Could you check a few things on this model? Use its own coordinates, in mm. A direction names the side the tool comes from. Round coordinates to 2 decimals unless told otherwise and drop trailing zeros. Loops run counter-clockwise (first coordinate to the right, second up) from the corner with the lowest first, then second, coordinate; pieces in that order, holes last.
Autodesk Inventor part; units mm, degrees
ref_plane "Plano de trabajo1" through (0, 91.5, 0) normal (0, 1, 0) x (1, 0, 0)
ref_plane "YZ Plane" through (0, 0, 0) normal (1, 0, 0) x (0, 1, 0)
ref_plane "XZ Plane" through (0, 0, 0) normal (0, 1, 0) x (-1, 0, 0)
sketch "Boceto1" plane through (0, 0, 0) normal (0, 1, 0) x (-1, 0, 0)
  circle A0 centre (0, 0) radius 11
  dimension "d0" = 22
extrude "Extrusión1" add sketch "Boceto1" along normal blind 105
ref_plane "Plano de trabajo1" through (0, 91.5, 0) normal (0, 1, 0) x (1, 0, 0)
sketch "Boceto2" plane through (0, 91.5, 0) normal (0, 1, 0) x (1, 0, 0)
  circle A0 centre (0, 0) radius 11
  circle A1 centre (0, 0) radius 10
  dimension "d4" = 20
extrude "Extrusión2" cut sketch "Boceto2" against normal blind 1
thread "Rosca1"
properties part number "W520superior"
Item 1: For faces 5 (the flat face through (2, 90.5, 10)), 6 (the cylindrical face through (2.38, 98.16, 10.74)), which set-ups out of +Z, -Z, +X, -X, +Y, -Y let a thin tool reach every point of the face, with its end or its side?
Results list:
face 5: none
face 6: +Y, -Y
Item 2: We'd pull the mould along Y, two halves only. Please class faces 1 (the flat face through (0, 0, 0)), 2 (the cylindrical face through (2.38, 44.62, 10.74)), 3 (the cylindrical face through (-2.17, 91.01, 9.76)), 4 (the flat face through (2, 91.5, 10)): released by +Y, released by -Y, zero draft, split by the parting line, or undercut.
Results list:
face 1: released by -Y
face 2: zero draft
face 3: undercut
face 4: undercut
Item 3: If we section it at A-A, the plane x = 7: Please give me the cut outline in (y, z).
Results list:
outline: (0, -8.49) - (90.5, -8.49) - (90.5, -7.14) - (91.5, -7.14) - (91.5, -8.49) - (105, -8.49) - (105, 8.49) - (91.5, 8.49) - (91.5, 7.14) - (90.5, 7.14) - (90.5, 8.49) - (0, 8.49) - close
Item 4: If we section it at C-C, the plane y = 40.5: Please give me the cut outline in (x, z).
Results list:
outline: circle Ø22 at (0, 0)
Item 5: If we section it at B-B, the plane z = -3.75: Please give me the cut outline in (x, y), then the cut area to 3 significant figures.
Results list:
outline: (-10.34, 0) - (10.34, 0) - (10.34, 90.5) - (9.27, 90.5) - (9.27, 91.5) - (10.34, 91.5) - (10.34, 105) - (-10.34, 105) - (-10.34, 91.5) - (-9.27, 91.5) - (-9.27, 90.5) - (-10.34, 90.5) - close
area: 2,170 mm2
Item 6: If I drill on line 1 along Z through (x, y) = (-1.5, 79); line 2 along Z through (x, y) = (0, 24); line 3 along X through (y, z) = (63, 10), over which ranges is the centre line in solid material (lowest first)?
Results list:
line 1: z = -10.9 to 10.9
line 2: z = -11 to 11
line 3: x = -4.58 to 4.58
Item 7: Will these pins go through, and if not, where does the flat tip stop? pin 1 (1 mm diameter, centred on y = 73.5, z = -7, fed in from -X); pin 2 (1.5 mm diameter, centred on y = 49, z = 8.5, fed in from +X); pin 3 (2 mm diameter, centred on x = -8, y = 18.5, fed in from +Z).
Results list:
pin 1: stops at x = -8.87
pin 2: stops at x = 7.81
pin 3: stops at z = 8.49
